The model under review builds one solid part; all positions refer to its coordinate system, in mm. Face numbers are marked on the shaded views. A direction names the side the tool comes from. Coordinates: 2 decimals unless noted, no trailing zeros. Order: outer loops, then holes, each group sorted by start corner. A loop starts at its lowest first (then second) coordinate and runs counter-clockwise, first axis right, second up. Notation, with made-up numbers: M 71.5,84 L 95.5,84 A7 ccw 95.5,88 Z; hole C 53.5,2 d6. An arc over 180 degrees is marked long. Answer in a Markdown table with one row per item.
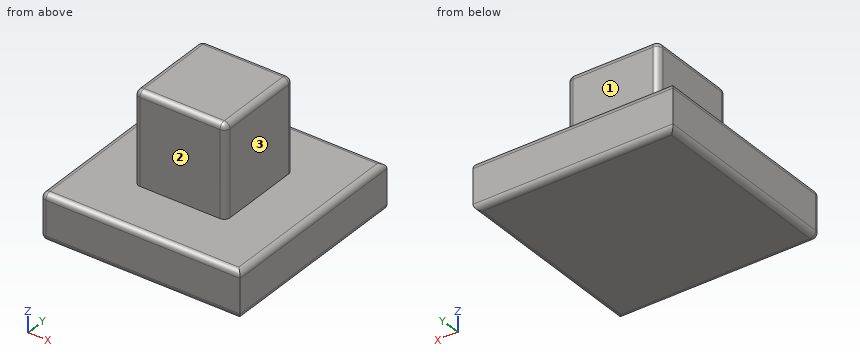
from build123d import *

# Parameters (mm, degrees)
F0_W     = 174.909296
F0_H     = 174.909296
F1_DEPTH = 40
F2_DEPTH = 120
F3_R     = 5


with BuildPart() as f1:
    # F0 (on Top) → F1 (new body)
    with BuildSketch(Plane.XY):
        Rectangle(F0_W, F0_H)
        Polygon((40, -40), (0, -40), (-40, -40), (-40, 40), (40, 40), align=None, mode=Mode.SUBTRACT)
    extrude(amount=F1_DEPTH)

    # F0 (on Top) → F2 (join)
    with BuildSketch(Plane.XY):
        Polygon((-40, -40), (0, -40), (40, -40), (40, 40), (-40, 40), align=None)
    extrude(amount=F2_DEPTH)

    # F3
    f3_edges = [f1.edges().sort_by_distance(p)[0] for p in [
        (0, -40, 120),
        (40, 0, 120),
        (-40, 0, 120),
        (0, 40, 120),
        (40, 40, 80),
        (40, -40, 80),
        (-40, -40, 80),
        (-40, 40, 80),
        (-87.454648, 0, 40),
        (0, -87.454648, 40),
        (0, -87.454648, 0),
        (-87.454648, 0, 0),
        (-87.454648, -87.454648, 20),
        (87.454648, 0, 40),
        (87.454648, 0, 0),
        (0, 87.454648, 0),
        (0, 87.454648, 40),
    ]]
    fillet(f3_edges, radius=F3_R)


solid = f1.part
(1) Machinability: for the marked faces 1, 2 and 3, which of the approach directions +Z, -Z, +X, -X, +Y, -Y give a long, thin tool a straight path to every point of the face, cutting with its end or side? Answer none if there is none.
Report:
| item | result |
|---|---|
| face 1 | +Z, +X, -X, +Y |
| face 2 | +Z, +X, -X, -Y |
| face 3 | +Z, +X, +Y, -Y |
(2) Insertion check: P1, Ø10, axis at y = 33.5, z = 83, coming from the +X side; P2, Ø6, axis at y = 23, z = 49, coming from the -X side; P3, Ø2, axis at x = 31.5, y = 36.5, coming from the +Z side. Each pin has a flat end and moves straight along its axis. Give the tip position at first contact, or say it passes through.
Report:
| item | result |
|---|---|
| P1 | x = 40 |
| P2 | x = -40 |
| P3 | z = 119.97 |
(3) To check wall thickness, follow line 1 (Z direction, x = 60.5, y = 40); line 2 (X direction, y = -6, z = 41). State the ranges of each line that lie inside material, in increasing order. Write a range as [from, to].
Report:
| item | result |
|---|---|
| line 1 | [0, 40] |
| line 2 | [-40, 40] |
(4) Take a section at B-B (z = 80). Write out the cut boundary in (x, y).
Report:
| item | result |
|---|---|
| outline | M -40,-35 A5 ccw -35,-40 L 35,-40 A5 ccw 40,-35 L 40,35 A5 ccw 35,40 L -35,40 A5 ccw -40,35 Z |
(5) Take a section at C-C (y = 6). Write out the cut boundary in (x, z).
Report:
| item | result |
|---|---|
| outline | M -87.45,5 A5 ccw -82.45,0 L 82.45,0 A5 ccw 87.45,5 L 87.45,35 A5 ccw 82.45,40 L 40,40 L 40,115 A5 ccw 35,120 L -35,120 A5 ccw -40,115 L -40,40 L -82.45,40 A5 ccw -87.45,35 Z |
(6) Take a section at A-A (x = -74.5). Write out the cut boundary in (y, z), then the cut area to 3 significant figures.
Report:
| item | result |
|---|---|
| outline | M -87.45,5 A5 ccw -82.45,0 L 82.45,0 A5 ccw 87.45,5 L 87.45,35 A5 ccw 82.45,40 L -82.45,40 A5 ccw -87.45,35 Z |
| area | 6,970 mm^2 |
